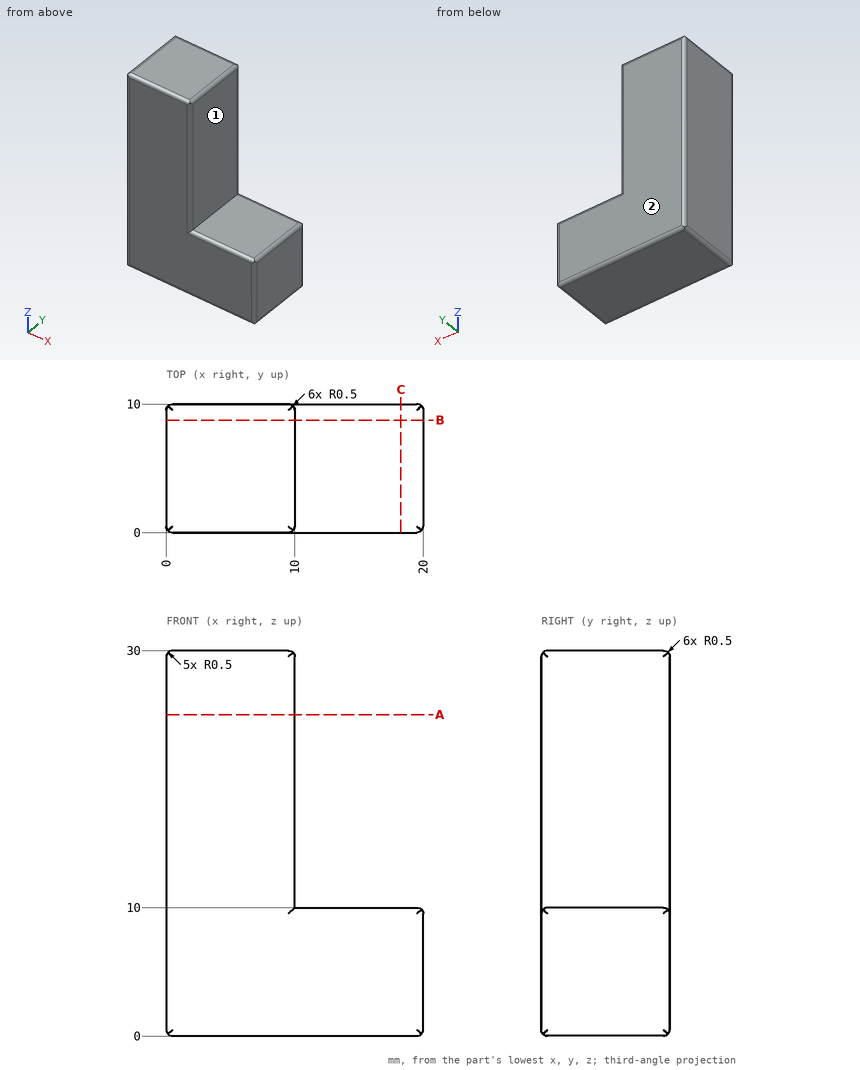
Check sheet for the drawn part. Datum: minimum x, y, z corner. Units: mm. A direction names the side the tool comes from. Give positions to 0.01 mm unless a question says otherwise; leave off trailing zeros. Order: outer loops, then holes, each group sorted by start corner. A loop starts at its lowest first (then second) coordinate and runs counter-clockwise, first axis right, second up. Notation, with made-up numbers: (48, 12.5) -> (93, 12.5) arc R31 cw to (93, 48.5) -> close; hole circle Ø8 at (12, -8). An arc over 180 degrees is marked (long way). Use a Markdown table: item, result.
1) Tool access check on the marked faces 1 and 2. Record the directions out of +Z, -Z, +X, -X, +Y, -Y that give a thin tool (end or side, any length) a straight path to the whole face; none if there is none.
Results:
| item | result |
|---|---|
| face 1 | +Z, +X, +Y, -Y |
| face 2 | +Z, -Z, +X, -X, +Y |
2) Material ranges on probe 1 along Z at (x, y) = (14.25, 7); probe 2 along Z at (x, y) = (14, 9.75), recorded low to high.
Results:
| item | result |
|---|---|
| probe 1 | 0 to 10 |
| probe 2 | 0.07 to 9.93 |
3) Depth check by flat-ended pin: pin 1 Ø2.5 at (y, z) = (4.5, 15.5) entering from +X; pin 2 Ø10 at (x, z) = (11.5, 11.5) entering from +Y. Enter the tip coordinate at first touch or a pass-through.
Results:
| item | result |
|---|---|
| pin 1 | x = 10 |
| pin 2 | y = 10 |
4) Section check A-A, the plane z = 25. Record the boundary of the cut face in (x, y).
Results:
| item | result |
|---|---|
| outline | (0, 0.5) arc R0.5 ccw to (0.5, 0) -> (9.5, 0) arc R0.5 ccw to (10, 0.5) -> (10, 9.5) arc R0.5 ccw to (9.5, 10) -> (0.5, 10) arc R0.5 ccw to (0, 9.5) -> close |
5) Section check B-B, the plane y = 8.75. Record the boundary of the cut face in (x, z).
Results:
| item | result |
|---|---|
| outline | (0, 0.5) arc R0.5 ccw to (0.5, 0) -> (19.5, 0) arc R0.5 ccw to (20, 0.5) -> (20, 9.5) arc R0.5 ccw to (19.5, 10) -> (10, 10) -> (10, 29.5) arc R0.5 ccw to (9.5, 30) -> (0.5, 30) arc R0.5 ccw to (0, 29.5) -> close |
